from build123d import *

# Parameters (mm, degrees)
F1_DEPTH = 6.35
F2_R     = 5.08


with BuildPart() as f1:
    # F0 (on Front) → F1 (new body, symmetric)
    with BuildSketch(Plane.XZ):
        with BuildLine():
            Line((-133.693446, -48.976308), (-117.367371, -60.302993))
            Line((-117.367371, -60.302993), (84.090313, -60.302993))
            Line((84.090313, -60.302993), (140.153468, -27.65083))
            Line((140.153468, -27.65083), (117.05051, -27.65083))
            Line((117.05051, -27.65083), (80.435061, -48.976308))
            Line((80.435061, -48.976308), (36.960306, -48.976308))
            ThreePointArc((36.960306, -48.976308), (-3.347569, -17.650078), (4.924222, 32.724866))
            Line((4.924222, 32.724866), (91.518199, 32.724866))
            Line((91.518199, 32.724866), (91.518199, 38.724854))
            Line((91.518199, 38.724854), (73.902904, 38.724854))
            Line((73.902904, 38.724854), (73.902904, 44.494075))
            Line((73.902904, 44.494075), (63.902899, 44.494075))
            Line((63.902899, 44.494075), (63.902899, 38.494087))
            Line((63.902899, 38.494087), (-49.86607, 38.494087))
            Line((-49.86607, 38.494087), (-49.86607, 44.724842))
            Line((-49.86607, 44.724842), (-59.866076, 44.724842))
            Line((-59.866076, 44.724842), (-59.866076, 38.724854))
            Line((-59.866076, 38.724854), (-92.173692, 38.724854))
            Line((-92.173692, 38.724854), (-92.173692, 32.724866))
            Line((-92.173692, 32.724866), (-1.852643, 32.724866))
            ThreePointArc((-1.852643, 32.724866), (-11.856696, -14.771434), (22.581745, -48.976308))
            Line((22.581745, -48.976308), (-133.693446, -48.976308))
        make_face()
    extrude(amount=F1_DEPTH, both=True)

    # F2
    f2_edges = [f1.edges().sort_by_distance(p)[0] for p in [
        (22.581745, 0, -48.976308),
        (-1.852643, 0, 32.724866),
    ]]
    fillet(f2_edges, radius=F2_R)


solid = f1.part
Read the model definition and answer for the solid it produces. Units are mm, in the model's axes. A direction names the side the tool comes from. Round coordinates to 2 decimals unless told otherwise and drop trailing zeros. Write each loop counter-clockwise with the first axis right and the second up, starting at its lowest first coordinate (ties: lowest second). Pieces come first, ordered by that corner, then holes. Notation, with made-up numbers: M -23.5,-23.75 L -16.5,-23.75 A32 cw -16.5,3.25 Z; hole C 0,-19 d9. An arc over 180 degrees is marked long. Use a Markdown table: item, result.
1) For a pull along X with two mould halves and no side action, classify faces 6 (the flat face through (48, 0, 32.725)), 7 (the flat face through (59, 0, -48.976)), 8 (the flat face through (91.518, 0, 36)) as pulls with the +X half, pulls with the -X half, needs draft (parallel to the pull), parting line crosses it, or undercut.
Answers follow:
| item | result |
|---|---|
| face 6 | needs draft |
| face 7 | undercut |
| face 8 | pulls with the +X half |
2) The part is cut by section A-A (x = 47.5). Write down the section's boundary in (y, z), plus the area to 3 significant figures.
Answers follow:
| item | result |
|---|---|
| outline | M -6.35,-60.3 L 6.35,-60.3 L 6.35,-48.98 L -6.35,-48.98 Z; M -6.35,32.72 L 6.35,32.72 L 6.35,38.49 L -6.35,38.49 Z |
| area | 217 mm2 |
3) Flat-ended cylindrical pins translate along their axes: pin 1 (6.5 mm diameter, centred on y = 3, z = 40.5, fed in from -X); pin 2 (2 mm diameter, centred on y = 3.5, z = -0.5, fed in from +X); pin 3 (2 mm diameter, centred on x = -74.5, y = -1, fed in from +Z). Find the tip coordinate at first contact, or state that the pin passes through.
Answers follow:
| item | result |
|---|---|
| pin 1 | stops at x = -92.17 |
| pin 2 | stops at x = -6.75 |
| pin 3 | stops at z = 38.72 |
4) Straight lines are drawn through the part: line 1 along Z through (x, y) = (-45, 0.75); line 2 along Z through (x, y) = (-60, 2.5); line 3 along Z through (x, y) = (-103.5, 2.75). For each, find the intervals that lie inside material, in ascending order. Write a range as [from, to].
Answers follow:
| item | result |
|---|---|
| line 1 | z = [-60.3, -48.98], [32.72, 38.49] |
| line 2 | z = [-60.3, -48.98], [32.72, 38.72] |
| line 3 | z = [-60.3, -48.98] |
5) The part is cut by section D-D (x = -98). Write down the section's boundary in (y, z), plus the area to 3 significant figures.
Answers follow:
| item | result |
|---|---|
| outline | M -6.35,-60.3 L 6.35,-60.3 L 6.35,-48.98 L -6.35,-48.98 Z |
| area | 144 mm2 |
6) A tool of negligible diameter and unlimited length cuts with its end or side. For faces 1 (the flat face through (129, 0, -27.651)), 2 (the flat face through (-65, 0, -48.976)), 3 (the cylindrical face through (-3.068, -0.089, -18.346)), 4 (the flat face through (-59.866, 0, 42)), 5 (the flat face through (-49.866, 0, 42)), from which of +Z, -Z, +X, -X, +Y, -Y can it reach the whole face along a straight path? Write none if from no direction.
Answers follow:
| item | result |
|---|---|
| face 1 | +Z, +X, +Y, -Y |
| face 2 | -X, +Y, -Y |
| face 3 | +Y, -Y |
| face 4 | +Z, -X, +Y, -Y |
| face 5 | +Z, +Y, -Y |
7) The part is cut by section C-C (y = 0.75). Write down the section's boundary in (x, z).
Answers follow:
| item | result |
|---|---|
| outline | M -133.69,-48.98 L -117.37,-60.3 L 84.09,-60.3 L 140.15,-27.65 L 117.05,-27.65 L 80.44,-48.98 L 36.96,-48.98 A49.94 cw 4.92,32.72 L 91.52,32.72 L 91.52,38.72 L 73.9,38.72 L 73.9,44.49 L 63.9,44.49 L 63.9,38.49 L -49.87,38.49 L -49.87,44.72 L -59.87,44.72 L -59.87,38.72 L -92.17,38.72 L -92.17,32.72 L -11.62,32.72 A5.08 cw -7.22,25.11 A50.79 ccw 5.13,-39.92 A5.08 cw 1.97,-48.98 Z |
8) The part is cut by section B-B (z = -46). Write down the section's boundary in (x, y), plus the area to 3 significant figures.
Answers follow:
| item | result |
|---|---|
| outline | M 6.59,-6.35 L 25.14,-6.35 L 25.14,6.35 L 6.59,6.35 Z; M 85.55,-6.35 L 108.65,-6.35 L 108.65,6.35 L 85.55,6.35 Z |
| area | 529 mm2 |
